Verification items for this drawing (mm, ordinates from the low corner). A direction names the side the tool comes from. Round coordinates to 2 decimals unless told otherwise and drop trailing zeros. Loops run counter-clockwise (first coordinate to the right, second up) from the corner with the lowest first, then second, coordinate; pieces in that order, holes last. Notation, with made-up numbers: M 52,-35.75 L 64,-35.75 A18 ccw 64,-1.75 Z; hole C -11.5,82 d11. An arc over 180 degrees is marked long. Write item = value, one per line. Start each with the question number.
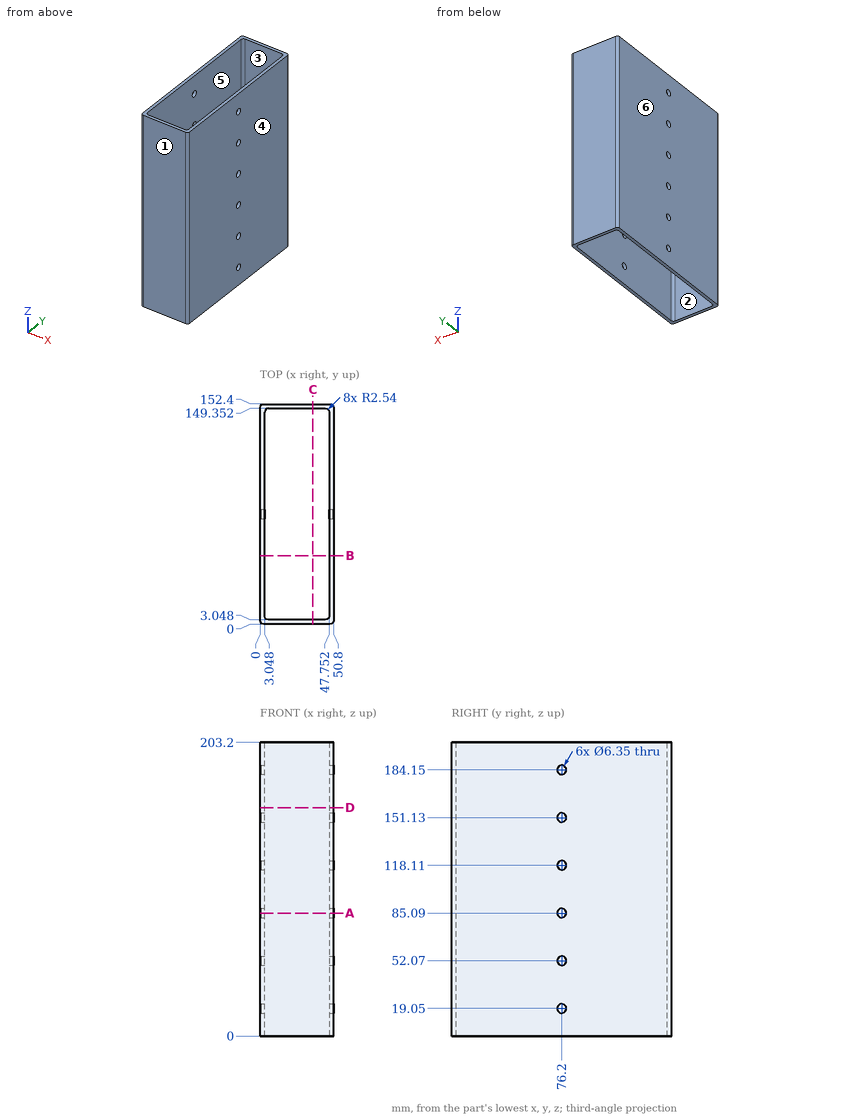
1. Section check A-A, the plane z = 85.09. Enter the section's corners in (x, y) (3 decimals).
2. Section check B-B, the plane y = 47.5. Enter the section's corners in (x, z), and give its area (3 significant figures).
3. Tool access check on the marked faces 5 and 6. Record the directions out of +Z, -Z, +X, -X, +Y, -Y that give a thin tool (end or side, any length) a straight path to the whole face; none if there is none.
4. Gauge pin test, flat end, axial feed: P1, Ø4, axis at y = 76.2, z = 151.13, coming from the -X side. Record the tip position at first contact, or that the pin passes through.
5. Mould release check, pull along X, two halves, no side actions. Record for the marked faces 1, 2, 3 and 4: pulls with the +X half, pulls with the -X half, needs draft (parallel to the pull), parting line crosses it, or undercut.
6. Thickness scan on line 1 (X direction, y = 133, z = 66); line 2 (Y direction, x = 21, z = 81); line 3 (Y direction, x = 48.5, z = 179). Record the ranges inside material, lowest first.
7. Section check C-C, the plane x = 36.5. Enter the section's corners in (y, z).
8. Section check D-D, the plane z = 158. Enter the section's corners in (x, y).
Computed values:
q1.outline = M 0,2.54 A2.54 ccw 2.54,0 L 48.26,0 A2.54 ccw 50.8,2.54 L 50.8,73.025 L 47.752,73.025 L 47.752,5.588 A2.54 cw 45.212,3.048 L 5.588,3.048 A2.54 cw 3.048,5.588 L 3.048,73.025 L 0,73.025 Z; M 0,79.375 L 3.048,79.375 L 3.048,146.812 A2.54 cw 5.588,149.352 L 45.212,149.352 A2.54 cw 47.752,146.812 L 47.752,79.375 L 50.8,79.375 L 50.8,149.86 A2.54 ccw 48.26,152.4 L 2.54,152.4 A2.54 ccw 0,149.86 Z
q2.outline = M 0,0 L 3.05,0 L 3.05,203.2 L 0,203.2 Z; M 47.75,0 L 50.8,0 L 50.8,203.2 L 47.75,203.2 Z
q2.area = 1,240 mm2
q3.face_5 = +Z, -Z
q3.face_6 = +Z, -Z, -X, +Y, -Y
q4.P1 = through
q5.face_1 = needs draft
q5.face_2 = undercut
q5.face_3 = undercut
q5.face_4 = pulls with the +X half
q6.line_1 = 0 to 3.05, 47.75 to 50.8
q6.line_2 = 0 to 3.05, 149.35 to 152.4
q6.line_3 = 0.01 to 152.39
q7.outline = M 0,0 L 3.05,0 L 3.05,203.2 L 0,203.2 Z; M 149.35,0 L 152.4,0 L 152.4,203.2 L 149.35,203.2 Z
q8.outline = M 0,2.54 A2.54 ccw 2.54,0 L 48.26,0 A2.54 ccw 50.8,2.54 L 50.8,149.86 A2.54 ccw 48.26,152.4 L 2.54,152.4 A2.54 ccw 0,149.86 Z; hole M 3.05,5.59 A2.54 ccw 5.59,3.05 L 45.21,3.05 A2.54 ccw 47.75,5.59 L 47.75,146.81 A2.54 ccw 45.21,149.35 L 5.59,149.35 A2.54 ccw 3.05,146.81 Z
